from build123d import *

# Parameters (mm, degrees)
SKETCH1_W           = 300
SKETCH1_H           = 209.332
SKETCH1_R           = 25
SKETCH1_R_2         = 27.5
SKETCH1_R_3         = 25.5
SKETCH1_W_2         = 55
SKETCH1_H_2         = 55
SKETCH1_W_3         = 51
SKETCH1_H_3         = 51
SKETCH1_W_4         = 50
SKETCH1_H_4         = 50
BOSS_EXTRUDE1_DEPTH = 10
SKETCH2_W           = 50
SKETCH2_H           = 50
CUT_EXTRUDE1_DEPTH  = 1
BOSS_EXTRUDE2_START = -9
SKETCH3_R           = 25
BOSS_EXTRUDE2_DEPTH = 8
SKETCH4_W           = 50
SKETCH4_H           = 50
CUT_EXTRUDE2_DEPTH  = 366.950660915
FILLET1_R           = 10
SKETCH5_W           = 50
SKETCH5_H           = 50
BOSS_EXTRUDE3_DEPTH = 10
SKETCH6_R           = 25
SKETCH6_W           = 50
SKETCH6_H           = 50
CUT_EXTRUDE3_DEPTH  = 366.950660915
BOSS_EXTRUDE4_START = -1
SKETCH7_W           = 50
SKETCH7_H           = 50
BOSS_EXTRUDE4_DEPTH = 9
SKETCH8_R           = 25
CUT_EXTRUDE4_DEPTH  = 1


with BuildPart() as part:
    # Sketch1 → Boss-Extrude1 (new body)
    with BuildSketch(Plane(origin=(0, 0, 0), x_dir=(1, 0, 0), z_dir=(0, 1, 0))):
        with Locations((150, 104.666)):
            Rectangle(SKETCH1_W, SKETCH1_H)
        with Locations(Location((45, 156.999, 0), (0, 0, 270))):
            Circle(SKETCH1_R, mode=Mode.SUBTRACT)
        with Locations(Location((45, 52.333, 0), (0, 0, 270))):
            Circle(SKETCH1_R, mode=Mode.SUBTRACT)
        with Locations(Location((115, 156.999, 0), (0, 0, 270))):
            Circle(SKETCH1_R_2, mode=Mode.SUBTRACT)
        with Locations(Location((185, 156.999, 0), (0, 0, 270))):
            Circle(SKETCH1_R_3, mode=Mode.SUBTRACT)
        with Locations(Location((255, 156.999, 0), (0, 0, 270))):
            Circle(SKETCH1_R, mode=Mode.SUBTRACT)
        with Locations((115, 52.333)):
            Rectangle(SKETCH1_W_2, SKETCH1_H_2, mode=Mode.SUBTRACT)
        with Locations((185, 52.333)):
            Rectangle(SKETCH1_W_3, SKETCH1_H_3, mode=Mode.SUBTRACT)
        with Locations((255, 52.333)):
            Rectangle(SKETCH1_W_4, SKETCH1_H_4, mode=Mode.SUBTRACT)
    extrude(amount=BOSS_EXTRUDE1_DEPTH)

    # Sketch2 → Cut-Extrude1 (cut)
    with BuildSketch(Plane(origin=(0, 10, 0), x_dir=(1, 0, 0), z_dir=(0, 1, 0))):
        with Locations((45, 156.999)):
            Rectangle(SKETCH2_W, SKETCH2_H)
    extrude(amount=-CUT_EXTRUDE1_DEPTH, mode=Mode.SUBTRACT)

    # Sketch3 → Boss-Extrude2 (add)
    with BuildSketch(Plane(origin=(0, 9, 0), x_dir=(1, 0, 0), z_dir=(0, 1, 0)).offset(BOSS_EXTRUDE2_START)):
        with Locations(Location((45, 156.999, 0), (0, 0, 270))):
            Circle(SKETCH3_R)
    extrude(amount=BOSS_EXTRUDE2_DEPTH)

    # Sketch4 → Cut-Extrude2 (cut, through all)
    with BuildSketch(Plane(origin=(0, 10, 0), x_dir=(1, 0, 0), z_dir=(0, 1, 0))):
        with Locations((45, 52.333)):
            Rectangle(SKETCH4_W, SKETCH4_H)
    extrude(amount=-CUT_EXTRUDE2_DEPTH, mode=Mode.SUBTRACT)

    # Fillet1
    fillet1_edges = [part.edges().sort_by_distance(p)[0] for p in [
        (0, 5, -209.332),
        (300, 5, -209.332),
        (300, 5, 0),
        (0, 5, 0),
    ]]
    fillet(fillet1_edges, radius=FILLET1_R)

    # Sketch5 → Boss-Extrude3 (add)
    with BuildSketch(Plane(origin=(0, 10, 0), x_dir=(1, 0, 0), z_dir=(0, 1, 0))):
        with Locations((45, 156.999)):
            Rectangle(SKETCH5_W, SKETCH5_H)
        with Locations((45, 52.333)):
            Rectangle(SKETCH5_W, SKETCH5_H)
    extrude(amount=-BOSS_EXTRUDE3_DEPTH)

    # Sketch6 → Cut-Extrude3 (cut, through all)
    with BuildSketch(Plane(origin=(0, 10, 0), x_dir=(1, 0, 0), z_dir=(0, 1, 0))):
        with Locations(Location((43.75, 105, 0), (0, 0, 270))):
            Circle(SKETCH6_R)
        with Locations((43.75, 40)):
            Rectangle(SKETCH6_W, SKETCH6_H)
        with Locations((43.75, 170)):
            Rectangle(SKETCH6_W, SKETCH6_H)
    extrude(amount=-CUT_EXTRUDE3_DEPTH, mode=Mode.SUBTRACT)

    # Sketch7 → Boss-Extrude4 (add)
    with BuildSketch(Plane(origin=(0, 10, 0), x_dir=(1, 0, 0), z_dir=(0, 1, 0)).offset(BOSS_EXTRUDE4_START)):
        with Locations((43.75, 170)):
            Rectangle(SKETCH7_W, SKETCH7_H)
    extrude(amount=-BOSS_EXTRUDE4_DEPTH)

    # Sketch8 → Cut-Extrude4 (cut)
    with BuildSketch(Plane(origin=(0, 9, 0), x_dir=(1, 0, 0), z_dir=(0, 1, 0))):
        with Locations(Location((43.75, 170, 0), (0, 0, 270))):
            Circle(SKETCH8_R)
    extrude(amount=-CUT_EXTRUDE4_DEPTH, mode=Mode.SUBTRACT)


solid = part.part
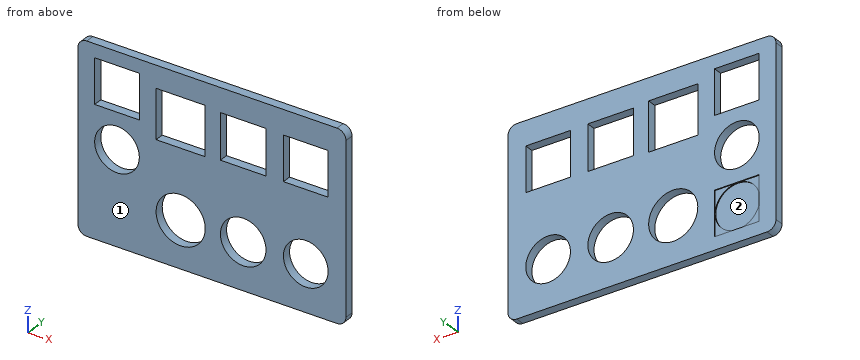
For this review, take the finished solid that the model builds, in its own axes (mm). Face numbers are marked on the shaded views. Give positions to 0.01 mm unless a question says otherwise; leave off trailing zeros. Order: outer loops, then holes, each group sorted by start corner. A loop starts at its lowest first (then second) coordinate and runs counter-clockwise, first axis right, second up. Notation, with made-up numbers: (30.25, 36) - (44.25, 36) arc R21 cw to (44.25, 68) - close; hole circle Ø9 at (71, 85.5). An arc over 180 degrees is marked (long way). Answer as a JSON object with one key per item and string values. Group by question number.
Item 1: Take a section at C-C on z = -32.5. Give the boundary of the cut face in (x, y).
Item 2: Wall thickness on line 1 along X through (y, z) = (1, -32); line 2 along X through (y, z) = (9.25, -74.5); line 3 along X through (y, z) = (4.5, -105): over which ranges is each line inside the solid? List them lowest first.
Item 3: Take a section at D-D on z = -105. Give the boundary of the cut face in (x, y), and give its area (3 significant figures).
Item 4: Take a section at A-A on x = 255. Give the boundary of the cut face in (y, z).
Item 5: Clearance check with a flat-ended pin moving along its axis: pin 1 Ø7.5 at (x, z) = (52, -184.5) entering from +Y. State where the tip first meets the part, or that it passes through.
Item 6: Take a section at B-B on y = 3. Give the number of separate pieces and of enclosed holes in the cut face, and give its area (3 significant figures).
Item 7: Draft analysis for pull direction Z (two halves, no side actions). For the marked faces 1 and 2, state which applies: pulls with the +Z half, pulls with the -Z half, needs draft (parallel to the pull), parting line crosses it, or undercut.
Reported:
{
 "1": {"outline": "(0, 0) - (18.75, 0) - (18.75, 10) - (0, 10) - close; (68.75, 0) - (87.5, 0) - (87.5, 10) - (68.75, 10) - close; (142.5, 0) - (159.5, 0) - (159.5, 10) - (142.5, 10) - close; (210.5, 0) - (230, 0) - (230, 10) - (210.5, 10) - close; (280, 0) - (300, 0) - (300, 10) - (280, 10) - close"},
 "2": {"line 1": "0 to 18.75, 68.75 to 87.5, 142.5 to 159.5, 210.5 to 230, 280 to 300", "line 2": "0 to 87.5, 142.5 to 159.5, 210.5 to 230, 280 to 300", "line 3": "0 to 18.75, 68.75 to 300"},
 "3": {"outline": "(0, 0) - (18.75, 0) - (18.75, 10) - (0, 10) - close; (68.75, 0) - (300, 0) - (300, 10) - (68.75, 10) - close", "area": "2,500 mm^2"},
 "4": {"outline": "(0, -209.33) - (10, -209.33) - (10, -182) - (0, -182) - close; (0, -132) - (10, -132) - (10, -77.33) - (0, -77.33) - close; (0, -27.33) - (10, -27.33) - (10, 0) - (0, 0) - close"},
 "5": {"pin 1": "y = 8"},
 "6": {"separate pieces": "1", "enclosed holes": "8", "area": "43,700 mm^2"},
 "7": {"face 1": "needs draft", "face 2": "undercut"}
}
